The listing builds one solid part. Answer for the finished solid, in the listing's coordinates (mm). A direction names the side the tool comes from. Coordinates: 2 decimals unless noted, no trailing zeros. Use one line per item in the form item = value. Start each with the question number.
```python
from build123d import *

# Parameters (mm, degrees)
F1_DEPTH = 50.8
F2_R     = 3.99999


# Not quite as in the source:
# - a fillet or chamfer is up to 0.001 mm smaller than in the source, because OpenCascade refuses the exact size


with BuildPart() as f1:
    # F0 (on Front) → F1 (new body)
    with BuildSketch(Plane.XZ):
        Polygon((71.5625, 0), (0, 0), (0, -50.8), (8, -50.8), (8, -8), (63.5625, -8), (63.5625, -84.2), (114.3625, -84.2), (114.3625, -58.8), (106.3625, -58.8), (106.3625, -76.2), (71.5625, -76.2), align=None)
    extrude(amount=F1_DEPTH)

    # F2 (radius 4 in the source; OpenCascade refuses exactly that, so slightly less here)
    f2_edges = [f1.edges().sort_by_distance(p)[0] for p in [
        (0, -25.4, 0),
        (71.5625, -25.4, 0),
        (71.5625, -25.4, -76.2),
        (106.3625, -25.4, -76.2),
        (71.5625, -50.8, -38.1),
        (71.5625, 0, -38.1),
        (110.3625, 0, -58.8),
        (114.3625, -25.4, -58.8),
        (110.3625, -50.8, -58.8),
        (106.3625, -25.4, -58.8),
        (114.3625, -25.4, -84.2),
        (114.3625, -50.8, -71.5),
        (114.3625, 0, -71.5),
        (88.9625, 0, -84.2),
        (88.9625, -50.8, -84.2),
        (63.5625, -25.4, -84.2),
        (63.5625, -50.8, -46.1),
        (63.5625, 0, -46.1),
        (0, 0, -25.4),
        (0, -50.8, -25.4),
        (0, -25.4, -50.8),
        (88.9625, 0, -76.2),
        (8, 0, -29.4),
        (8, -50.8, -29.4),
        (35.78125, -50.8, -8),
        (88.9625, -50.8, -76.2),
        (106.3625, 0, -67.5),
        (4, -50.8, -50.8),
        (106.3625, -50.8, -67.5),
        (8, -25.4, -50.8),
        (35.78125, -50.8, 0),
        (35.78125, 0, 0),
        (8, -25.4, -8),
        (63.5625, -25.4, -8),
        (4, 0, -50.8),
        (35.78125, 0, -8),
    ]]
    fillet(f2_edges, radius=F2_R)


solid = f1.part
```
(1) Find the intervals of material crossed by probe 1 along X at (y, z) = (-23, -25); probe 2 along X at (y, z) = (-49, -75.5); probe 3 along Z at (x, y) = (94.5, -15), in increasing order. Write a range as from..to.
(2) For faces 1 (the face through (9.141, -25.7, -9.203)), 2 (the face through (88.775, -49.597, -77.341)), 3 (the face through (6.859, -49.597, -29.156)), 4 (the face through (6.859, -1.203, -29.156)), 5 (the face through (72.765, -25.7, -75.059)), determine the directions among +Z, -Z, +X, -X, +Y, -Y from which every point of the face is accessible in a straight line to the end or side of a thin tool.
(3) Determine the mould class of faces 6 (the face through (89.262, -1.203, -83.059)), 7 (the face through (36.114, -49.597, -6.859)), 8 (the face through (113.22, -49.6, -71.38)) for opening direction X: +X half, -X half, draft (parallel to the pull), parting line (faces both ways), or undercut.
(4) Each of these flat-tipped pins is pushed along its axis until it touches: pin 1 Ø8 at (x, y) = (93.5, -35) entering from +Z; pin 2 Ø3 at (y, z) = (-36, -66.5) entering from -X; pin 3 Ø4 at (y, z) = (-28, -36) entering from +X. Where does it stop, or does it pass through?
Evaluation:
q1.probe_1 = 0..8, 63.56..71.56
q1.probe_2 = 64.22..72.27, 105.65..113.7
q1.probe_3 = -84.2..-76.2
q2.face_1 = -Z, +Y, -Y
q2.face_2 = +Z, -Y
q2.face_3 = -Z, -Y
q2.face_4 = -Z, +Y
q2.face_5 = +Z, +Y, -Y
q3.face_6 = draft
q3.face_7 = undercut
q3.face_8 = +X half
q4.pin_1 = -76.2
q4.pin_2 = 63.56
q4.pin_3 = 71.56
